```python
from build123d import *

# Parameters (mm, degrees)
REVOLVE_1_ANGLE          = 40
SKETCH_3_W               = 5.2
SKETCH_3_H               = 5.2
CUT_EXTRUDE_1_DEPTH      = 7
CUT_EXTRUDE_2_DEPTH      = 94.967026614
CUT_EXTRUDE_2_DEPTH_BACK = 94.967026614
SKETCH_5_R               = 1.5
CUT_EXTRUDE_START        = -2
SKETCH_6_R               = 3
CUT_EXTRUDE_3_DEPTH      = 93.938324905
SKETCH_12_R              = 1.5
CUT_EXTRUDE_5_DEPTH      = 54.141615619
CUT_EXTRUDE_6_DEPTH      = 5
SKETCH_14_W              = 3
SKETCH_14_H              = 3
PATTERN_CIRCULAR_1_COUNT = 4
PATTERN_CIRCULAR_1_ANGLE = 15
F_1_THE_OTHER_WAY_COUNT  = 4
F_1_THE_OTHER_WAY_ANGLE  = 15
SKETCH_9_W               = 1.8
SKETCH_9_H               = 4.8
SKETCH_9_H_2             = 2.8
EXTRUDE_2_DEPTH          = 3
SKETCH_10_W              = 52.448370613
SKETCH_10_H              = 39.953744926
CUT_EXTRUDE_4_DEPTH      = 149.179341739
SKETCH_11_W              = 14
SKETCH_11_H              = 30
EXTRUDE_3_DEPTH          = 5
FILLET_1_R               = 5


# Read off the part's stored shape, not the designer's step: 旋转1
with BuildPart() as part:
    # 旋转1 outline → 旋转1 (revolve)
    with BuildSketch(Plane(origin=(0, 0, 0), x_dir=(0.3420201433256701, 0, -0.9396926207859079), z_dir=(0.9396926207859079, 0, 0.3420201433256701))):
        Polygon((134, 5), (125, 5), (125, -5), (134, -5), (134, -7.5), (136.5, -10), (139, -7.5), (139, 7.5), (136.5, 10), (134, 7.5), align=None)
    revolve(axis=Axis((0, 0, 0), (0, 1, 0)), revolution_arc=REVOLVE_1_ANGLE)

    # 草图3 → 切除-拉伸1 (cut)
    with BuildSketch(Plane(origin=(0, 0, 0), x_dir=(0.34202014332566943, 0, -0.9396926207859081), z_dir=(0.9396926207859081, 0, 0.34202014332566943))):
        with Locations((132, 0)):
            Rectangle(SKETCH_3_W, SKETCH_3_H)
    extrude(amount=-CUT_EXTRUDE_1_DEPTH, mode=Mode.SUBTRACT)

    # 草图5 → 切除-拉伸2 (cut, two sides: drawn at the far end of the back side and taken through both)
    with BuildSketch(Plane(origin=(44.257406546, 0, -121.59622513), x_dir=(-0.9396926207859081, 0, -0.3420201433256695), z_dir=(0.3420201433256695, 0, -0.9396926207859081)).offset(-CUT_EXTRUDE_2_DEPTH_BACK)):
        with Locations((3.5, 0)):
            Circle(SKETCH_5_R)
    extrude(amount=CUT_EXTRUDE_2_DEPTH + CUT_EXTRUDE_2_DEPTH_BACK, mode=Mode.SUBTRACT)

    # 草图6 → 切除-拉伸3 (cut, through all)
    with BuildSketch(Plane(origin=(46.035911292, 0, -126.482626758), x_dir=(0.9396926207859081, 0, 0.3420201433256695), z_dir=(-0.3420201433256695, 0, 0.9396926207859081)).offset(CUT_EXTRUDE_START)):
        with Locations((-3.5, 0)):
            Circle(SKETCH_6_R)
    extrude(amount=-CUT_EXTRUDE_3_DEPTH, mode=Mode.SUBTRACT)

    # 草图12 → 切除-拉伸5 (cut, through all)
    with BuildSketch(Plane(origin=(0, 0, -139), x_dir=(-1, 0, 0), z_dir=(0, 0, -1))):
        Circle(SKETCH_12_R)
    cut_extrude_5 = extrude(amount=-CUT_EXTRUDE_5_DEPTH, mode=Mode.SUBTRACT)

    # 草图13 → 切除-拉伸6 (cut)
    with BuildSketch(Plane(origin=(0, 0, -139), x_dir=(-1, 0, 0), z_dir=(0, 0, -1))):
        Polygon((0, -3.175426481), (2.75, -1.58771324), (2.75, 1.58771324), (0, 3.175426481), (-2.75, 1.58771324), (-2.75, -1.58771324), align=None)
    cut_extrude_6 = extrude(amount=-CUT_EXTRUDE_6_DEPTH, mode=Mode.SUBTRACT)

    # 草图14 → 切除-旋转1 (revolve, cut)
    with BuildSketch(Plane(origin=(0, 0, 0), x_dir=(1, 0, 0), z_dir=(0, 1, 0)), mode=Mode.PRIVATE) as cut_revolve_1_sk:
        with Locations((1.5, 126.463994814)):
            Rectangle(SKETCH_14_W, SKETCH_14_H)
    cut_revolve_1 = revolve(cut_revolve_1_sk.sketch.rotate(Axis((0, 0, 1000), (0, 0, -1)), 180), axis=Axis((0, 0, 1000), (0, 0, -1)), mode=Mode.SUBTRACT)

    # 阵列(圆周)1: 切除-拉伸5, 切除-拉伸6, 切除-旋转1 ×4 about axis
    pattern_circular_1_axis = Axis((0, 0, 0), (0, 1, 0))
    add([cut_extrude_5.rotate(pattern_circular_1_axis, i * PATTERN_CIRCULAR_1_ANGLE / (PATTERN_CIRCULAR_1_COUNT - 1)) for i in range(1, PATTERN_CIRCULAR_1_COUNT)], mode=Mode.SUBTRACT)
    add([cut_extrude_6.rotate(pattern_circular_1_axis, i * PATTERN_CIRCULAR_1_ANGLE / (PATTERN_CIRCULAR_1_COUNT - 1)) for i in range(1, PATTERN_CIRCULAR_1_COUNT)], mode=Mode.SUBTRACT)
    add([cut_revolve_1.rotate(pattern_circular_1_axis, i * PATTERN_CIRCULAR_1_ANGLE / (PATTERN_CIRCULAR_1_COUNT - 1)) for i in range(1, PATTERN_CIRCULAR_1_COUNT)], mode=Mode.SUBTRACT)

    # 1 the other way: 切除-拉伸5, 切除-拉伸6, 切除-旋转1 ×4 about axis
    f_1_the_other_way_axis = Axis((0, 0, 0), (0, -1, 0))
    add([cut_extrude_5.rotate(f_1_the_other_way_axis, i * F_1_THE_OTHER_WAY_ANGLE / (F_1_THE_OTHER_WAY_COUNT - 1)) for i in range(1, F_1_THE_OTHER_WAY_COUNT)], mode=Mode.SUBTRACT)
    add([cut_extrude_6.rotate(f_1_the_other_way_axis, i * F_1_THE_OTHER_WAY_ANGLE / (F_1_THE_OTHER_WAY_COUNT - 1)) for i in range(1, F_1_THE_OTHER_WAY_COUNT)], mode=Mode.SUBTRACT)
    add([cut_revolve_1.rotate(f_1_the_other_way_axis, i * F_1_THE_OTHER_WAY_ANGLE / (F_1_THE_OTHER_WAY_COUNT - 1)) for i in range(1, F_1_THE_OTHER_WAY_COUNT)], mode=Mode.SUBTRACT)

    # 草图9 → 凸台-拉伸2 (add)
    with BuildSketch(Plane(origin=(0, 0, 0), x_dir=(0.34202014332566943, 0, -0.9396926207859082), z_dir=(0.9396926207859082, 0, 0.34202014332566943))):
        with Locations((138.1, 0)):
            Rectangle(SKETCH_9_W, SKETCH_9_H)
        with Locations((125.9, 3.6)):
            Rectangle(SKETCH_9_W, SKETCH_9_H_2)
        with Locations((125.9, -3.6)):
            Rectangle(SKETCH_9_W, SKETCH_9_H_2)
    extrude(amount=EXTRUDE_2_DEPTH)

    # 草图10 → 切除-拉伸4 (cut, through all)
    with BuildSketch(Plane(origin=(0, 0, 0), x_dir=(0, -1, 0), z_dir=(0.9990482215818578, 0, -0.04361938736533606))):
        with Locations((1.816079314, 125.001454628)):
            Rectangle(SKETCH_10_W, SKETCH_10_H)
    extrude(amount=-CUT_EXTRUDE_4_DEPTH, mode=Mode.SUBTRACT)

    # 草图11 → 凸台-拉伸3 (add)
    with BuildSketch(Plane(origin=(0, 0, 0), x_dir=(0.043619387365336076, 0, 0.9990482215818578), z_dir=(-0.9990482215818577, 0, 0.04361938736533607))):
        with Locations((-132, 0)):
            Rectangle(SKETCH_11_W, SKETCH_11_H)
    extrude(amount=EXTRUDE_3_DEPTH)

    # 圆角1
    fillet_1_edges = [part.edges().sort_by_distance(p)[0] for p in [
        (-8.560715398, 15, -138.758654331),
        (-8.560715398, -15, -138.758654331),
        (-7.950043975, -15, -124.771979229),
        (-7.950043975, 15, -124.771979229),
    ]]
    fillet(fillet_1_edges, radius=FILLET_1_R)


solid = part.part
```
Here's how the part is built. I have some questions about the finished solid (model axes, mm). A direction names the side the tool comes from. Give positions to 0.01 mm unless a question says otherwise; leave off trailing zeros. Write each loop counter-clockwise with the first axis right and the second up, starting at its lowest first coordinate (ties: lowest second). Pieces come first, ordered by that corner, then holes. Notation, with made-up numbers: M -14,20.5 L 0,20.5 A20 cw 0,41.5 Z; hole C 6.5,18 d3. An arc over 180 degrees is marked long. Put each result on its own line as item: value. Start each with the question number.
Item 1: If we section it at B-B, the plane y = -11: Write out the boundary of the cut face in (x, z).
Item 2: Thinking about a two-plate mould opening in Y: for faces 6 (the flat face through (20, 5, -127)), 7 (the flat face through (-8.53, -0.14, -138.76)), 8 (the flat face through (36.65, 2.39, -131.53)), which applies, +Y half, -Y half, draft (parallel to the pull), parting line (faces both ways), or undercut?
Item 3: I need wall thicknesses on L1, parallel to Y at x = 45, z = -118; L2, parallel to Y at x = 0, z = -132; L3, parallel to X at y = 0, z = -137. Which ranges of each line are inside material? Lowest first, please. Write a range as from..to.
Item 4: On a 3-axis mill with a long thin cutter (end or side, diameter ignored), from which of +Z, -Z, +X, -X, +Y, -Y can I reach the whole of each face in a straight line? I mean faces 1 (the flat face through (22.336, 2.37, -134.703)), 2 (the flat face through (44.142, 3.58, -116.956)), 3 (the flat face through (38, 0, -131.2)), 4 (the flat face through (-7.915, -0.14, -124.774)), 5 (the flat face through (44.758, -3.62, -118.647)). Say none if no direction works.
Item 5: If we section it at A-A, the plane y = 0: Count the separate pieces of the cut face and the enclosed holes in it, then the cut area to 3 significant figures.
Item 6: Will these pins go through, and if not, where does the flat tip stop? pin 1 (12 mm diameter, centred on x = 37, y = -8.5, fed in from +Z); pin 2 (1.6 mm diameter, centred on x = 1, y = 1, fed in from -Z); pin 3 (5 mm diameter, centred on x = -1, y = 1, fed in from +Z); pin 4 (6 mm diameter, centred on x = -3.5, z = -128.5, fed in from -Y).
Values:
1. outline: M -11.05,-138.55 L -6.06,-138.77 L -5.46,-124.98 L -10.45,-124.76 Z
2. face 6: +Y half
2. face 7: draft
2. face 8: undercut
3. L1: -5..-2.2, 2.2..5
3. L2: -5..-1.5, 1.5..5
3. L3: -10.99..-2.75, 2.75..9.23, 14.75..21.36
4. face 1: none
4. face 2: +Z, -X, +Y, -Y
4. face 3: -Z
4. face 4: +Z, +Y, -Y
4. face 5: +X, +Y, -Y
5. separate pieces: 7
5. enclosed holes: 0
5. area: 478 mm²
6. pin 1: z = -117.78
6. pin 2: z = -134
6. pin 3: z = -124.95
6. pin 4: y = -15
